Geometry check sheet. Reference: drawing and pictorial views, mm from the part's lowest x, y, z. A direction names the side the tool comes from. Round coordinates to 2 decimals unless told otherwise and drop trailing zeros. Write each loop counter-clockwise with the first axis right and the second up, starting at its lowest first coordinate (ties: lowest second). Pieces come first, ordered by that corner, then holes. Notation, with made-up numbers: (-17.75, -39.5) - (15.25, -39.5) arc R31 ccw to (15.25, -2.5) - close; hole circle Ø1 at (47, 6). An arc over 180 degrees is marked (long way). Return JSON: item names as keys, results as strings.
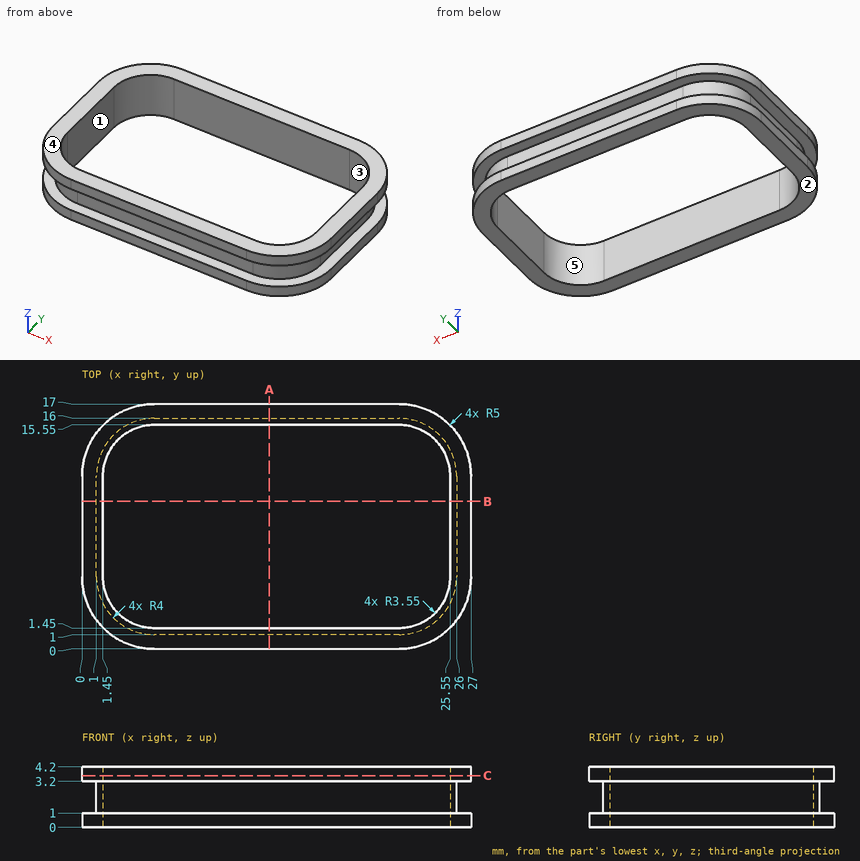
(1) Release check for a two-part mould opening along Y. For the marked faces 1, 2 and 3 record: pulls with the +Y half, pulls with the -Y half, needs draft (parallel to the pull), parting line crosses it, or undercut.
Response values:
{"face 1": "undercut", "face 2": "needs draft", "face 3": "undercut"}
(2) Access from +Z, -Z, +X, -X, +Y, -Y to the whole of each face (thin tool, end or side, straight path). Record for the marked faces 4 and 5.
Response values:
{"face 4": "+Z, +X, -X, +Y, -Y", "face 5": "+Z, -Z"}
(3) Section check A-A, the plane x = 13. Enter the section's corners in (y, z).
Response values:
{"outline": "(0, 0) - (1.45, 0) - (1.45, 4.2) - (0, 4.2) - (0, 3.2) - (1, 3.2) - (1, 1) - (0, 1) - close; (15.55, 0) - (17, 0) - (17, 1) - (16, 1) - (16, 3.2) - (17, 3.2) - (17, 4.2) - (15.55, 4.2) - close"}
(4) Gauge pin test, flat ends, axial feed: pin 1 (1.1 mm diameter, centred on y = 8.5, z = 2, fed in from -X); pin 2 (1 mm diameter, centred on x = 7.5, z = 2.5, fed in from +Y); pin 3 (1.8 mm diameter, centred on x = 10, z = 2, fed in from -Y). Record the tip position at first contact, or that the pin passes through.
Response values:
{"pin 1": "stops at x = 1", "pin 2": "stops at y = 16", "pin 3": "stops at y = 1"}
(5) Material ranges on line 1 along Y through (x, z) = (7.25, 1.95); line 2 along Y through (x, z) = (6.5, 4.05); line 3 along X through (y, z) = (8.25, 1.75), recorded low to high. Write a range as [from, to].
Response values:
{"line 1": "y = [1, 1.45], [15.55, 16]", "line 2": "y = [0, 1.45], [15.55, 17]", "line 3": "x = [1, 1.45], [25.55, 26]"}
(6) Section check C-C, the plane z = 3.6. Enter the section's corners in (x, y).
Response values:
{"outline": "(0, 5) arc R5 ccw to (5, 0) - (22, 0) arc R5 ccw to (27, 5) - (27, 12) arc R5 ccw to (22, 17) - (5, 17) arc R5 ccw to (0, 12) - close; hole (1.45, 5) arc R3.55 ccw to (5, 1.45) - (22, 1.45) arc R3.55 ccw to (25.55, 5) - (25.55, 12) arc R3.55 ccw to (22, 15.55) - (5, 15.55) arc R3.55 ccw to (1.45, 12) - close"}
(7) Section check B-B, the plane y = 10.25. Enter the section's corners in (x, z), plus the area to 3 significant figures.
Response values:
{"outline": "(0, 0) - (1.45, 0) - (1.45, 4.2) - (0, 4.2) - (0, 3.2) - (1, 3.2) - (1, 1) - (0, 1) - close; (25.55, 0) - (27, 0) - (27, 1) - (26, 1) - (26, 3.2) - (27, 3.2) - (27, 4.2) - (25.55, 4.2) - close", "area": "7.78 mm^2"}
